```python
from build123d import *

# Parameters (mm, degrees)
SKETCH1_R           = 76.2
SKETCH1_W           = 15
SKETCH1_H           = 5
SKETCH1_W_2         = 5
SKETCH1_H_2         = 15
BOSS_EXTRUDE1_DEPTH = 5


with BuildPart() as part:
    # Sketch1 → Boss-Extrude1 (new body)
    with BuildSketch(Plane(origin=(0, 0, 0), x_dir=(1, 0, 0), z_dir=(0, 1, 0))):
        with Locations(Location((0, 0, 0), (0, 0, 270))):
            Circle(SKETCH1_R)
        with Locations((0, 65.5)):
            Rectangle(SKETCH1_W, SKETCH1_H, mode=Mode.SUBTRACT)
        with Locations((-65.5, 0)):
            Rectangle(SKETCH1_W_2, SKETCH1_H_2, mode=Mode.SUBTRACT)
        with Locations((65.5, 0)):
            Rectangle(SKETCH1_W_2, SKETCH1_H_2, mode=Mode.SUBTRACT)
        with Locations((0, -65.5)):
            Rectangle(SKETCH1_W, SKETCH1_H, mode=Mode.SUBTRACT)
    extrude(amount=BOSS_EXTRUDE1_DEPTH)


solid = part.part
```
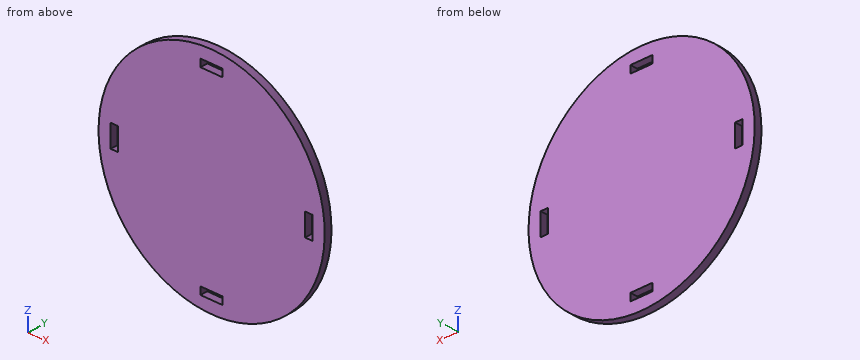
Design review of the part built by this model. Coordinates are the model's own, in mm. Coordinates: 2 decimals unless noted, no trailing zeros. Loops run counter-clockwise (first coordinate to the right, second up) from the corner with the lowest first, then second, coordinate; pieces in that order, holes last. Notation, with made-up numbers: (50, -6) -> (88, -6) arc R20 cw to (88, 24) -> close; hole circle Ø8 at (58, 70.5). An arc over 180 degrees is marked (long way). Answer as a JSON object with one key per item and string values.
Q1. Take a section at B-B on x = 0. Give the boundary of the cut face in (y, z), plus the area to 3 significant figures.
Answer block:
{"outline": "(0, -76.2) -> (5, -76.2) -> (5, -68) -> (0, -68) -> close; (0, -63) -> (5, -63) -> (5, 63) -> (0, 63) -> close; (0, 68) -> (5, 68) -> (5, 76.2) -> (0, 76.2) -> close", "area": "712 mm^2"}
Q2. Take a section at A-A on z = 0. Give the boundary of the cut face in (x, y), plus the area to 3 significant figures.
Answer block:
{"outline": "(-76.2, 0) -> (-68, 0) -> (-68, 5) -> (-76.2, 5) -> close; (-63, 0) -> (63, 0) -> (63, 5) -> (-63, 5) -> close; (68, 0) -> (76.2, 0) -> (76.2, 5) -> (68, 5) -> close", "area": "712 mm^2"}
Q3. Take a section at D-D on x = -27.5. Give the boundary of the cut face in (y, z), plus the area to 3 significant figures.
Answer block:
{"outline": "(0, -71.06) -> (5, -71.06) -> (5, 71.06) -> (0, 71.06) -> close", "area": "711 mm^2"}
Q4. To check wall thickness, follow L1, parallel to X at y = 1.3, z = 3; L2, parallel to Z at x = 4, y = 3.4; L3, parallel to X at y = 3.95, z = -65.5. State the ranges of each line that lie inside material, in increasing order.
Answer block:
{"L1": "x = -76.14 to -68, -63 to 63, 68 to 76.14", "L2": "z = -76.09 to -68, -63 to 63, 68 to 76.09", "L3": "x = -38.94 to -7.5, 7.5 to 38.94"}
Q5. Take a section at C-C on y = 1.5. Give the boundary of the cut face in (x, z).
Answer block:
{"outline": "circle Ø152.4 at (0, 0); hole (-68, -7.5) -> (-63, -7.5) -> (-63, 7.5) -> (-68, 7.5) -> close; hole (-7.5, -68) -> (7.5, -68) -> (7.5, -63) -> (-7.5, -63) -> close; hole (-7.5, 63) -> (7.5, 63) -> (7.5, 68) -> (-7.5, 68) -> close; hole (63, -7.5) -> (68, -7.5) -> (68, 7.5) -> (63, 7.5) -> close"}
Q6. Clearance check with flat-ended pins moving along their axes: pin 1 Ø2.5 at (y, z) = (3.5, 2) entering from +X; pin 2 Ø2.5 at (x, y) = (-1.5, 2) entering from +Z; pin 3 Ø1.5 at (y, z) = (3, -66.5) entering from -X. State where each tip first meets the part, or that it passes through.
Answer block:
{"pin 1": "stops at x = 76.2", "pin 2": "stops at z = 76.2", "pin 3": "stops at x = -38.51"}
